Part model, mm, in its own coordinate system. Face numbers are marked on the shaded views. A direction names the side the tool comes from. Coordinates: 2 decimals unless noted, no trailing zeros. Write each loop counter-clockwise with the first axis right and the second up, starting at its lowest first coordinate (ties: lowest second). Pieces come first, ordered by that corner, then holes. Notation, with made-up numbers: (62.25, 10.5) - (104.25, 10.5) arc R32 cw to (104.25, 38.5) - close; hole circle Ø1 at (23.5, 65.5). An arc over 180 degrees is marked (long way). Use a Markdown table: item, result.
```python
from build123d import *

# Parameters (mm, degrees)
SKETCH1_R           = 2
BOSS_EXTRUDE1_DEPTH = 40
SKETCH2_R           = 3.85
BOSS_EXTRUDE2_DEPTH = 3
FILLET1_R           = 1
FILLET2_R           = 1


with BuildPart() as part:
    # Sketch1 → Boss-Extrude1 (new body)
    with BuildSketch(Plane(origin=(0, 0, 0), x_dir=(1, 0, 0), z_dir=(0, 1, 0))):
        Circle(SKETCH1_R)
    extrude(amount=BOSS_EXTRUDE1_DEPTH)

    # Sketch2 → Boss-Extrude2 (add)
    with BuildSketch(Plane(origin=(0, 40, 0), x_dir=(1, 0, 0), z_dir=(0, 1, 0))):
        Circle(SKETCH2_R)
    extrude(amount=BOSS_EXTRUDE2_DEPTH)

    # Fillet1
    fillet1_edges = [part.edges().sort_by_distance(p)[0] for p in [
        (-3.85, 43, 0),
    ]]
    fillet(fillet1_edges, radius=FILLET1_R)

    # Fillet2
    fillet2_edges = [part.edges().sort_by_distance(p)[0] for p in [
        (-2, 0, 0),
        (-2, 40, 0),
    ]]
    fillet(fillet2_edges, radius=FILLET2_R)


solid = part.part
```
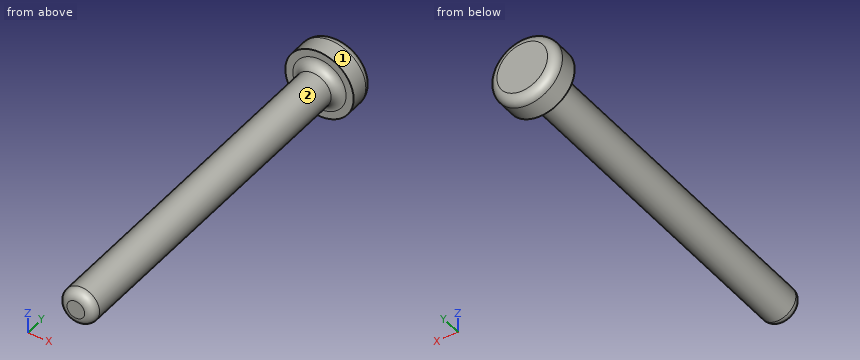
Item 1: Drill centre lines: probe 1 along X at (y, z) = (4.5, 1.75); probe 2 along Y at (x, z) = (-2.75, -0.5); probe 3 along Y at (x, z) = (1.75, 1.5). Where is each one in solid material? Low to high.
From the geometry:
| item | result |
|---|---|
| probe 1 | -0.97 to 0.97 |
| probe 2 | 39.98 to 43 |
| probe 3 | 39.72 to 43 |
Item 2: Drop flat-ended pins along their axis: P1, Ø1.5, axis at y = 5.5, z = -1, coming from the -X side; P2, Ø4, axis at x = 2.5, y = 27, coming from the -Z side; P3, Ø1, axis at y = 9.5, z = -3, coming from the -X side. Give the stop position or say it passes through.
From the geometry:
| item | result |
|---|---|
| P1 | x = -1.98 |
| P2 | z = -1.94 |
| P3 | through |
Item 3: Which spindle directions (+Z, -Z, +X, -X, +Y, -Y) get a long thin tool onto all of the face, cutting with end or side? Do the marked faces 1 and 2. Say none if no direction does.
From the geometry:
| item | result |
|---|---|
| face 1 | +Y, -Y |
| face 2 | -Y |
Item 4: Band-saw the part on A-A, the plane y = 35. Give the cut face in (x, z).
From the geometry:
| item | result |
|---|---|
| outline | circle Ø4 at (0, 0) |
